The listing builds one solid part. Answer for the finished solid, in the listing's coordinates (mm). Coordinates: 2 decimals unless noted, no trailing zeros. Order: outer loops, then holes, each group sorted by start corner. A loop starts at its lowest first (then second) coordinate and runs counter-clockwise, first axis right, second up. Notation, with made-up numbers: (43, -12.75) -> (95, -12.75) arc R19 cw to (95, -4.75) -> close; hole circle Ø5 at (54, 27.5). An arc over 180 degrees is marked (long way). Return JSON: item names as keys, results as strings.
```python
from build123d import *

# Parameters (mm, degrees)
SKETCH7_R           = 10
SKETCH7_R_2         = 19
BOSS_EXTRUDE7_DEPTH = 10


with BuildPart() as part:
    # Sketch7 → Boss-Extrude7 (new body)
    with BuildSketch(Plane(origin=(0, 0, 0), x_dir=(1, 0, 0), z_dir=(0, 1, 0))):
        with BuildLine():
            ThreePointArc((12.745045372, -105.413105413), (46.894193375, -46.39540437), (34.279777206, 20.61302682))
            ThreePointArc((34.279777206, 20.61302682), (1.47471049, 39.972806118), (-32.667709838, 23.082909998))
            ThreePointArc((-32.667709838, 23.082909998), (-36.445484769, 20.015963612), (-41.267553362, 19.363738157))
            ThreePointArc((-41.267553362, 19.363738157), (-63.99597338, 0.949285461), (-44.044461831, -20.442543154))
            Line((-44.044461831, -20.442543154), (-34.381716499, -20.442543154))
            ThreePointArc((-34.381716499, -20.442543154), (-27.977452206, -28.587797538), (-19.695904889, -34.814814815))
            ThreePointArc((-19.695904889, -34.814814815), (-6.734239862, -53.9492851), (-14.129670899, -75.845410628))
            ThreePointArc((-14.129670899, -75.845410628), (-14.800048672, -103.452083828), (12.745045372, -105.413105413))
        make_face()
        with Locations((-44.044461831, -0.442543154)):
            Circle(SKETCH7_R, mode=Mode.SUBTRACT)
        Circle(SKETCH7_R_2, mode=Mode.SUBTRACT)
        with Locations((0, -90)):
            Circle(SKETCH7_R, mode=Mode.SUBTRACT)
    extrude(amount=BOSS_EXTRUDE7_DEPTH)


solid = part.part
```
Item 1: Determine the mould class of faces 1 (the cylindrical face through (-52, 4.9, 6.5)), 2 (the flat face through (-39, 5, 20.443)), 3 (the cylindrical face through (8.767, 4.93, 16.856)), 4 (the cylindrical face through (-6.78, 4.93, 53.62)) for opening direction X: pulls with the +X half, pulls with the -X half, needs draft (parallel to the pull), parting line crosses it, or undercut.
Answer list:
{"face 1": "undercut", "face 2": "needs draft", "face 3": "undercut", "face 4": "pulls with the -X half"}
Item 2: The part is cut by section A-A on x = 0. Determine the outline of the cut face in (y, z), plus the area to 3 significant figures.
Answer list:
{"outline": "(0, -40) -> (10, -40) -> (10, -19) -> (0, -19) -> close; (0, 19) -> (10, 19) -> (10, 80) -> (0, 80) -> close; (0, 100) -> (10, 100) -> (10, 110) -> (0, 110) -> close", "area": "920 mm2"}
Item 3: The part is cut by section B-B on y = 5.75. Determine the outline of the cut face in (x, z).
Answer list:
{"outline": "(-44.04, 20.44) arc R20 ccw (long way) to (-41.27, -19.36) arc R9 cw to (-32.67, -23.08) arc R40 ccw to (34.28, -20.61) arc R98 ccw to (12.75, 105.41) arc R20 ccw to (-14.13, 75.85) arc R26 cw to (-19.7, 34.81) arc R40 ccw to (-34.38, 20.44) -> close; hole circle Ø20 at (-44.04, 0.44); hole circle Ø38 at (0, 0); hole circle Ø20 at (0, 90)"}
Item 4: The part is cut by section D-D on z = 38.5. Determine the outline of the cut face in (x, y).
Answer list:
{"outline": "(-14.69, 0) -> (47.92, 0) -> (47.92, 10) -> (-14.69, 10) -> close"}
Item 5: The part is cut by section C-C on z = 90. Determine the outline of the cut face in (x, y).
Answer list:
{"outline": "(-20, 0) -> (-10, 0) -> (-10, 10) -> (-20, 10) -> close; (10, 0) -> (27.69, 0) -> (27.69, 10) -> (10, 10) -> close"}
Item 6: Flat-ended cylindrical pins translate along their axes: pin 1 (1 mm diameter, centred on y = 2.5, z = 57, fed in from -X); pin 2 (6 mm diameter, centred on y = 5, z = -9, fed in from +X); pin 3 (3 mm diameter, centred on x = -38.5, y = 6.5, fed in from +Z). Find the tip coordinate at first contact, or state that the pin passes through.
Answer list:
{"pin 1": "x = -6.52", "pin 2": "x = 41.49", "pin 3": "z = 20.44"}
Item 7: Find the intervals of material crossed by probe 1 along Z at (x, y) = (0, 5); probe 2 along Z at (x, y) = (-17.5, 8.5); probe 3 along X at (y, z) = (8, -1.5), in increasing order.
Answer list:
{"probe 1": "-40 to -19, 19 to 80, 100 to 110", "probe 2": "-35.97 to -7.4, 7.4 to 36.21, 80.32 to 99.68", "probe 3": "-63.95 to -53.85, -34.23 to -18.94, 18.94 to 43.13"}
